Model file for the job. Use its own axes, mm. Face numbers are marked on the shaded views. A direction names the side the tool comes from. Give positions to 0.01 mm unless a question says otherwise; leave off trailing zeros. Order: outer loops, then holes, each group sorted by start corner. A loop starts at its lowest first (then second) coordinate and runs counter-clockwise, first axis right, second up. Notation, with made-up numbers: (16, 24.25) - (39, 24.25) arc R16 cw to (39, 38.25) - close; hole circle Ø7 at (60.25, -11.75). An arc over 180 degrees is marked (long way). Return JSON: item names as keys, results as strings. Group by question number.
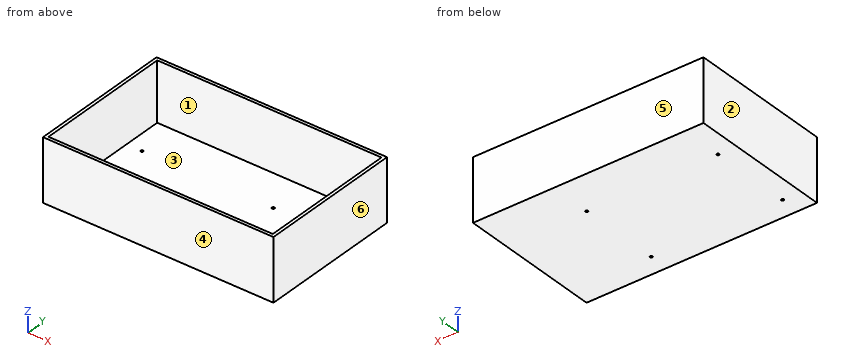
Autodesk Fusion 360 part; units mm, degrees
sketch "Sketch1" plane through (0, 0, 0) normal (0, 0, 1) x (1, 0, 0)
  line L0 (0, 0) -> (223, 0)
  line L1 (223, 0) -> (223, 140)
  line L2 (223, 140) -> (0, 140)
  line L3 (0, 140) -> (0, 0)
  dimension "d1" = 223
  dimension "d2" = 140
extrude "Extrude1" add sketch "Sketch1" along normal blind 60
sketch "Sketch2" plane through (0, 0, 60) normal (0, 0, 1) x (-1, 0, 0)
  line L0 (0, -140) -> (0, 0)
  line L1 (0, 0) -> (-223, 0)
  line L2 (-223, 0) -> (-223, -140)
  line L3 (-223, -140) -> (0, -140)
  line L4 (-3, -137) -> (-220, -137)
  line L5 (-220, -137) -> (-220, -3)
  line L6 (-220, -3) -> (-3, -3)
  line L7 (-3, -3) -> (-3, -137)
  dimension "d5" = 3
  dimension "d6" = 3
  dimension "d7" = 3
  dimension "d8" = 3
extrude "Extrude2" cut sketch "Sketch2" against normal blind 57 contours L4 L5 L6 L7
sketch "Sketch3" plane through (0, 0, 0) normal (0, 0, -1) x (1, 0, 0)
  line L0 (0, 0) -> (0, -140)
  line L1 (0, -140) -> (223, -140)
  line L2 (223, -140) -> (223, 0)
  line L3 (223, 0) -> (0, 0)
  line L4 (205.0199, -4.8072) -> (6.0134, -4.8072) construction
  line L5 (6.0134, -113.804) -> (205.0199, -113.804) construction
  line L6 (205.0199, -113.804) -> (9.7448, -113.804) construction
  line L7 (205.0199, -59.3055) -> (147.0519, -59.3055) construction
  circle A0 centre (145.0199, -99.104) radius 1.25
  circle A1 centre (145.0199, -19.507) radius 1.25
  circle A2 centre (18.0134, -99.104) radius 1.25
  line L8 (6.0134, -4.8072) -> (6.0134, -113.804) construction
  line L9 (205.0199, -113.804) -> (205.0199, -4.8072) construction
  line L10 (6.0134, -111.0749) -> (6.0134, -6.1412) construction
  circle A3 centre (18.0134, -19.507) radius 1.25
  point P0 (180.3238, -104.2905)
  dimension "d11" = 12
  dimension "d12" = 14.7
  dimension "d13" = 2.5
  dimension "d17" = 108.9968
  dimension "d18" = 54.4985
  dimension "d19" = 2.5
  dimension "d20" = 60
  dimension "d21" = 14.7
extrude "Extrude3" cut sketch "Sketch3" against normal up to surface (3 mm away) contours A0 | A1 | A2 | A3
(1) Slice it at A-A (z = 52). Give the cut face in (x, y), and give its area (3 significant figures).
(2) 3-axis set-ups, long thin cutter, end or side, ignore diameter. For the marked faces 1 and 2: which of +Z, -Z, +X, -X, +Y, -Y reach the whole face in a straight line?
(3) Slice it at B-B (x = 71.5). Give the cut face in (y, z).
(4) Pull direction Y, two halves, no side cores. Call the marked faces 3, 4, 5 and 6: released by +Y, released by -Y, zero draft, split by the parting line, or undercut.
(5) Drop a flat-ended pin along its axis: pin 1 Ø4 at (x, y) = (145.02, 99.1) entering from +Z. Give the stop position or say it passes through.
(6) Slice it at C-C (y = 89). Give the cut face in (x, z).
(7) Drill centre lines: L1, parallel to X at y = 119, z = 37; L2, parallel to Y at x = 37, z = 53.5; L3, parallel to Z at x = 186.5, y = 82. Where is each one in solid material? Low to high.
Result set:
{
 "1": {"outline": "(0, 0) - (223, 0) - (223, 140) - (0, 140) - close; hole (3, 3) - (220, 3) - (220, 137) - (3, 137) - close", "area": "2,140 mm²"},
 "2": {"face 1": "+Z", "face 2": "+Z, -Z, -X, +Y, -Y"},
 "3": {"outline": "(0, 0) - (140, 0) - (140, 60) - (137, 60) - (137, 3) - (3, 3) - (3, 60) - (0, 60) - close"},
 "4": {"face 3": "undercut", "face 4": "released by -Y", "face 5": "released by +Y", "face 6": "zero draft"},
 "5": {"pin 1": "stops at z = 3"},
 "6": {"outline": "(0, 0) - (223, 0) - (223, 60) - (220, 60) - (220, 3) - (3, 3) - (3, 60) - (0, 60) - close"},
 "7": {"L1": "x = 0 to 3, 220 to 223", "L2": "y = 0 to 3, 137 to 140", "L3": "z = 0 to 3"}
}
